Part print with two shaded views. Sizes in mm from the minimum x, y, z corner. Coordinates: 2 decimals unless noted, no trailing zeros. Loops run counter-clockwise (first coordinate to the right, second up) from the corner with the lowest first, then second, coordinate; pieces in that order, holes last.
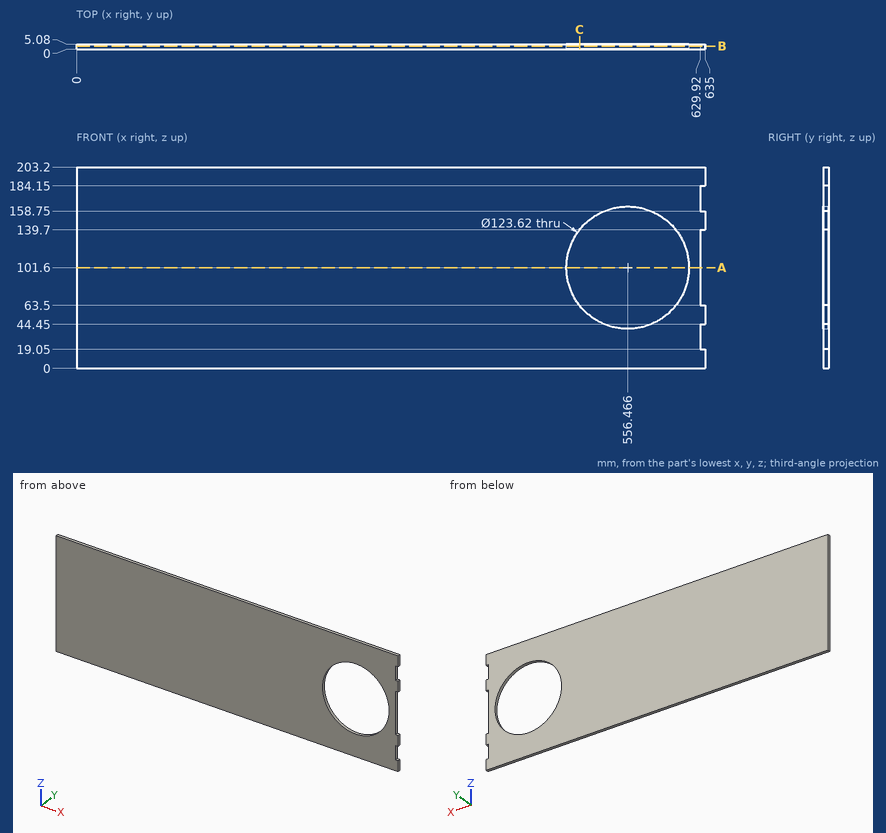
Q1. Slice it at A-A (z = 101.6). List the corners of the cut face in (x, y).
Answers:
outline: (0, 0) - (494.66, 0) - (494.66, 5.08) - (0, 5.08) - close; (618.28, 0) - (629.92, 0) - (629.92, 5.08) - (618.28, 5.08) - close
Q2. Slice it at C-C (x = 508). List the corners of the cut face in (y, z).
Answers:
outline: (0, 0) - (5.08, 0) - (5.08, 63.24) - (0, 63.24) - close; (0, 139.96) - (5.08, 139.96) - (5.08, 203.2) - (0, 203.2) - close
Q3. Drill centre lines: line 1 (X direction, y = 1.25, z = 101.6); line 2 (X direction, y = 0.9, z = 34); line 3 (Z direction, x = 561, y = 1). Where is each one in solid material? Low to high.
Answers:
line 1: x = 0 to 494.66, 618.28 to 629.92
line 2: x = 0 to 629.92
line 3: z = 0 to 39.96, 163.24 to 203.2
Q4. Flat gauge pins, fed straight in: P1, Ø2, axis at x = 350, z = 51.5, coming from the -Y side; P2, Ø2.5, axis at y = 1.5, z = 172, coming from the +X side. Where does each tip first touch, or does it go through?
Answers:
P1: stops at y = 0
P2: stops at x = 629.92
Q5. Slice it at B-B (y = 3). List the corners of the cut face in (x, z).
Answers:
outline: (0, 0) - (635, 0) - (635, 19.05) - (629.92, 19.05) - (629.92, 44.45) - (635, 44.45) - (635, 63.5) - (629.92, 63.5) - (629.92, 139.7) - (635, 139.7) - (635, 158.75) - (629.92, 158.75) - (629.92, 184.15) - (635, 184.15) - (635, 203.2) - (0, 203.2) - close; hole circle Ø123.62 at (556.47, 101.6)
